Design review of the part built by this model. Coordinates are the model's own, in mm. Face numbers are marked on the shaded views. Coordinates: 2 decimals unless noted, no trailing zeros. Order: outer loops, then holes, each group sorted by start corner. A loop starts at its lowest first (then second) coordinate and runs counter-clockwise, first axis right, second up. Notation, with made-up numbers: (55, -19.75) -> (91, -19.75) arc R19 cw to (91, 7.25) -> close; hole circle Ø5 at (86.5, 17). An arc over 180 degrees is marked (long way). Use a Markdown table: item, result. Add a question column.
Q1. Add section B-B (y = 20). State the section outline as (x, z) points (3 decimals).
Q2. Insertion check: pin 1 (4 mm diameter, centred on x = 12.5, y = -21.5, fed in from -Z). The pin has a flat end and moves straight along its axis. Give the tip position at first contact, or say it passes through.
Q3. Add section A-A (x = 35). State the section outline as (y, z) points (3 decimals).
Q4. The part is to be moulded in two halves that separate along Z. For the marked faces 1 and 2, say which applies: pulls with the +Z half, pulls with the -Z half, needs draft (parallel to the pull), parting line crosses it, or undercut.
Q5. Add section C-C (z = 2.3). State the section outline as (x, y) points (3 decimals), then the cut area to 3 significant figures.
Q6. Wall thickness on probe 1 along X at (y, z) = (4.5, 1.15) (3 decimals); probe 2 along Y at (x, z) = (-29, 0.25) (3 decimals); probe 3 along X at (y, z) = (-34, 0.8) (3 decimals): over which ranges is each line inside the solid? List them lowest first.
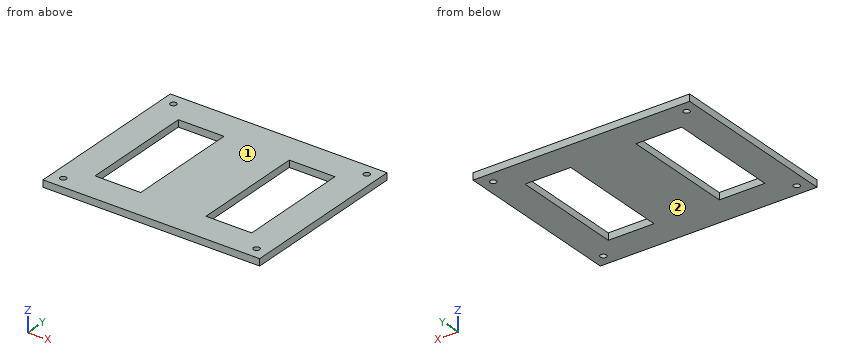
from build123d import *

# Parameters (mm, degrees)
SKETCH1_W           = 100.17
SKETCH1_H           = 80.17
BOSS_EXTRUDE1_DEPTH = 3.175
SKETCH3_R           = 1.415
CUT_EXTRUDE2_DEPTH  = 4.175
SKETCH2_W           = 21.13
SKETCH2_H           = 52.43
CUT_EXTRUDE4_DEPTH  = 10


with BuildPart() as part:
    # Sketch1 → Boss-Extrude1 (new body)
    with BuildSketch(Plane.XY):
        Rectangle(SKETCH1_W, SKETCH1_H)
    extrude(amount=BOSS_EXTRUDE1_DEPTH)

    # Sketch3 → Cut-Extrude2 (cut, through all)
    with BuildSketch(Plane.XY.offset(3.175)):
        with Locations((-44.696699141, 34.696699141)):
            Circle(SKETCH3_R)
        with Locations((44.696699141, 34.696699141)):
            Circle(SKETCH3_R)
        with Locations((44.696699141, -34.696699141)):
            Circle(SKETCH3_R)
        with Locations((-44.696699141, -34.696699141)):
            Circle(SKETCH3_R)
    extrude(amount=-CUT_EXTRUDE2_DEPTH, mode=Mode.SUBTRACT)

    # Sketch2 → Cut-Extrude4 (cut)
    with BuildSketch(Plane.XY.offset(3.175)):
        with Locations((25.65, 0)):
            Rectangle(SKETCH2_W, SKETCH2_H)
        with Locations((-25.65, 0)):
            Rectangle(SKETCH2_W, SKETCH2_H)
    extrude(amount=-CUT_EXTRUDE4_DEPTH, mode=Mode.SUBTRACT)


solid = part.part
Established:
| question | item | result |
|---|---|---|
| 1 | outline | (-50.085, 0) -> (-36.215, 0) -> (-36.215, 3.175) -> (-50.085, 3.175) -> close; (-15.085, 0) -> (15.085, 0) -> (15.085, 3.175) -> (-15.085, 3.175) -> close; (36.215, 0) -> (50.085, 0) -> (50.085, 3.175) -> (36.215, 3.175) -> close |
| 2 | pin 1 | z = 0 |
| 3 | outline | (-40.085, 0) -> (-26.215, 0) -> (-26.215, 3.175) -> (-40.085, 3.175) -> close; (26.215, 0) -> (40.085, 0) -> (40.085, 3.175) -> (26.215, 3.175) -> close |
| 4 | face 1 | pulls with the +Z half |
| 4 | face 2 | pulls with the -Z half |
| 5 | outline | (-50.085, -40.085) -> (50.085, -40.085) -> (50.085, 40.085) -> (-50.085, 40.085) -> close; hole circle Ø2.83 at (-44.697, -34.697); hole circle Ø2.83 at (-44.697, 34.697); hole (-36.215, -26.215) -> (-15.085, -26.215) -> (-15.085, 26.215) -> (-36.215, 26.215) -> close; hole (15.085, -26.215) -> (36.215, -26.215) -> (36.215, 26.215) -> (15.085, 26.215) -> close; hole circle Ø2.83 at (44.697, -34.697); hole circle Ø2.83 at (44.697, 34.697) |
| 5 | area | 5,790 mm^2 |
| 6 | probe 1 | -50.085 to -36.215, -15.085 to 15.085, 36.215 to 50.085 |
| 6 | probe 2 | -40.085 to -26.215, 26.215 to 40.085 |
| 6 | probe 3 | -50.085 to -45.928, -43.465 to 43.465, 45.928 to 50.085 |
